from build123d import *

# Parameters (mm, degrees)
BOSS_EXTRUDE1_DEPTH = 5
SKETCH3_R           = 20
CUT_EXTRUDE2_DEPTH  = 2
SKETCH4_R           = 2.5
BOSS_EXTRUDE2_DEPTH = 7
FILLET1_R           = 10


with BuildPart() as part:
    # Sketch1 → Boss-Extrude1 (new body)
    with BuildSketch(Plane.XY):
        with BuildLine():
            Line((-20, -40), (20, -40))
            ThreePointArc((20, -40), (34.142135624, -34.142135624), (40, -20))
            Line((40, -20), (40, 20))
            ThreePointArc((40, 20), (34.142135624, 34.142135624), (20, 40))
            Line((20, 40), (-20, 40))
            ThreePointArc((-20, 40), (-34.142135624, 34.142135624), (-40, 20))
            Line((-40, 20), (-40, -20))
            ThreePointArc((-40, -20), (-34.142135624, -34.142135624), (-20, -40))
        make_face()
    extrude(amount=BOSS_EXTRUDE1_DEPTH)

    # Sketch3 → Cut-Extrude2 (cut)
    with BuildSketch(Plane(origin=(0, 0, 0), x_dir=(-1, 0, 0), z_dir=(0, 0, -1))):
        Circle(SKETCH3_R)
    extrude(amount=-CUT_EXTRUDE2_DEPTH, mode=Mode.SUBTRACT)

    # Sketch4 → Boss-Extrude2 (add)
    with BuildSketch(Plane(origin=(0, 0, 2), x_dir=(-1, 0, 0), z_dir=(0, 0, -1))):
        Circle(SKETCH4_R)
        with BuildLine():
            Line((-0.997797575, 1.12), (-0.997797575, -1.12))
            ThreePointArc((-0.997797575, -1.12), (1.5, 0), (-0.997797575, 1.12))
        make_face(mode=Mode.SUBTRACT)
    extrude(amount=BOSS_EXTRUDE2_DEPTH)

    # Fillet1
    # the kernel refuses this fillet: 10 mm, written as the material it adds along each edge
    with BuildSketch(Plane(origin=(0, 0, 2), x_dir=(-1, 0, 0), z_dir=(0, -1, 0))) as fillet1_piece_1:
        with BuildLine():
            CenterArc((12.039392014, 10), FILLET1_R, 197.457603124, 72.542396876)
            Line((2.5, 7), (2.30921216, 6.94))
            ThreePointArc((2.30921216, 6.94), (2.3, 3.5), (2.3, 0))
            Line((2.3, 0), (2.5, -0.2))
            Line((2.5, -0.2), (12.039392014, -0.2))
            Line((12.039392014, -0.2), (12.039392014, 0))
        make_face()
    revolve(axis=Axis((0, 0, 2), (0, 0, -1)))


solid = part.part
Input: part model. Units: mm. Frame: model coordinates. A direction names the side the tool comes from. Coordinates: 2 decimals unless noted, no trailing zeros. Loops run counter-clockwise (first coordinate to the right, second up) from the corner with the lowest first, then second, coordinate; pieces in that order, holes last.
Q1. Material intervals for line 1 (Y direction, x = 0, z = 0.6); line 2 (Y direction, x = 0, z = 1.1); line 3 (Z direction, x = 36.5, y = 8), sorted ascending.
Q2. Cut plane B-B (x = 0). Output: boundary loops of the cut face in (y, z), then the cut area to 3 significant figures.
Q3. Set-up query: faces 1 (the face through (-9, -9, 2)), 2 (the face through (-33.986, 34.297, 2.465)). Return all of +Z, -Z, +X, -X, +Y, -Y with unobstructed straight access to the full face (end or side cutting, diameter ignored); none if empty.
Q4. Contact query for flat-ended pins moving along their axis: pin 1 (1.5 mm diameter, centred on y = -1, z = -3, fed in from +X); pin 2 (0.7 mm diameter, centred on x = -0.5, y = 0.5, fed in from -Z); pin 3 (10 mm diameter, centred on x = 31, y = -16.5, fed in from -Z). Output: stop coordinate, or through.
Q5. Cut plane D-D (y = 18). Output: boundary loops of the cut face in (x, z).
Q6. Cut plane A-A (z = 3.25). Output: boundary loops of the cut face in (x, y), then the cut area to 3 significant figures.
Q7. Cut plane C-C (y = 0). Output: boundary loops of the cut face in (x, z).
Q8. Draft query along Y for faces 3 (the face through (-34.297, -33.986, 2.465)), 4 (the face through (-1.5, 0, -1.5)), 5 (the face through (-9.4, 18.3, 0)). Return one class per face: +Y half, -Y half, draft (parallel to the pull), parting line (faces both ways), or undercut.
Working result:
1. line 1: y = -40 to -20, -6.94 to -1.5, 1.5 to 6.94, 20 to 40
1. line 2: y = -40 to -20, -7.89 to -1.5, 1.5 to 7.89, 20 to 40
1. line 3: z = 0 to 5
2. outline: (-40, 0) - (-20, 0) - (-20, 2) - (-12.04, 2) arc R10 cw to (-2.5, -5) - (-1.5, -5) - (-1.5, 2) - (1.5, 2) - (1.5, -5) - (2.5, -5) arc R10 cw to (12.04, 2) - (20, 2) - (20, 0) - (40, 0) - (40, 5) - (-40, 5) - close
2. area: 370 mm2
3. face 1: -Z
3. face 2: +Z, -Z, -X, +Y
4. pin 1: stops at x = 3.75
4. pin 2: stops at z = 2
4. pin 3: stops at z = 0
5. outline: (-40, 0) - (-8.72, 0) - (-8.72, 2) - (8.72, 2) - (8.72, 0) - (40, 0) - (40, 5) - (-40, 5) - close
6. outline: (-40, -20) arc R20 ccw to (-20, -40) - (20, -40) arc R20 ccw to (40, -20) - (40, 20) arc R20 ccw to (20, 40) - (-20, 40) arc R20 ccw to (-40, 20) - close
6. area: 6,060 mm2
7. outline: (-40, 0) - (-20, 0) - (-20, 2) - (-12.04, 2) arc R10 cw to (-2.5, -5) - (-1.5, -5) - (-1.5, 2) - (1, 2) - (1, -5) - (2.5, -5) arc R10 cw to (12.04, 2) - (20, 2) - (20, 0) - (40, 0) - (40, 5) - (-40, 5) - close
8. face 3: -Y half
8. face 4: undercut
8. face 5: draft
